Could you check a few things on this drawing? It's one solid part, dimensions in mm from its lowest x, y, z. A direction names the side the tool comes from. Round coordinates to 2 decimals unless told otherwise and drop trailing zeros. Loops run counter-clockwise (first coordinate to the right, second up) from the corner with the lowest first, then second, coordinate; pieces in that order, holes last. Notation, with made-up numbers: (53.25, 86.5) -> (83.25, 86.5) arc R36 cw to (83.25, 121.5) -> close; hole circle Ø11 at (25.5, 81.25). An arc over 180 degrees is marked (long way). Use one line per item in the form item = value. Start each with the question number.
Item 1: For the marked faces 1 and 2, which set-ups out of +Z, -Z, +X, -X, +Y, -Y let a thin tool reach every point of the face, with its end or its side?
Item 2: If I drill on L1, parallel to Z at x = 550, y = 694.5; L2, parallel to Z at x = 361, y = 277 (1 decimal); L3, parallel to Y at x = 428, z = 458 (1 decimal), over which ranges is the centre line in solid material (lowest first)? Write a range as [from, to].
Item 3: If we section it at B-B (z = 282.5): Write out the boundary of the cut face in (x, y) (1 decimal).
Item 4: I'm going to push flat-ended pins straight in: pin 1 Ø3 at (x, z) = (148, 293.5) entering from -Y (1 decimal); pin 2 Ø6 at (x, z) = (396, 549) entering from +Y; pin 3 Ø10 at (y, z) = (592, 236) entering from -X. Where does each tip first touch, or does it pass through?
Item 5: If we section it at A-A (z = 608): Write out the boundary of the cut face in (x, y) (1 decimal).
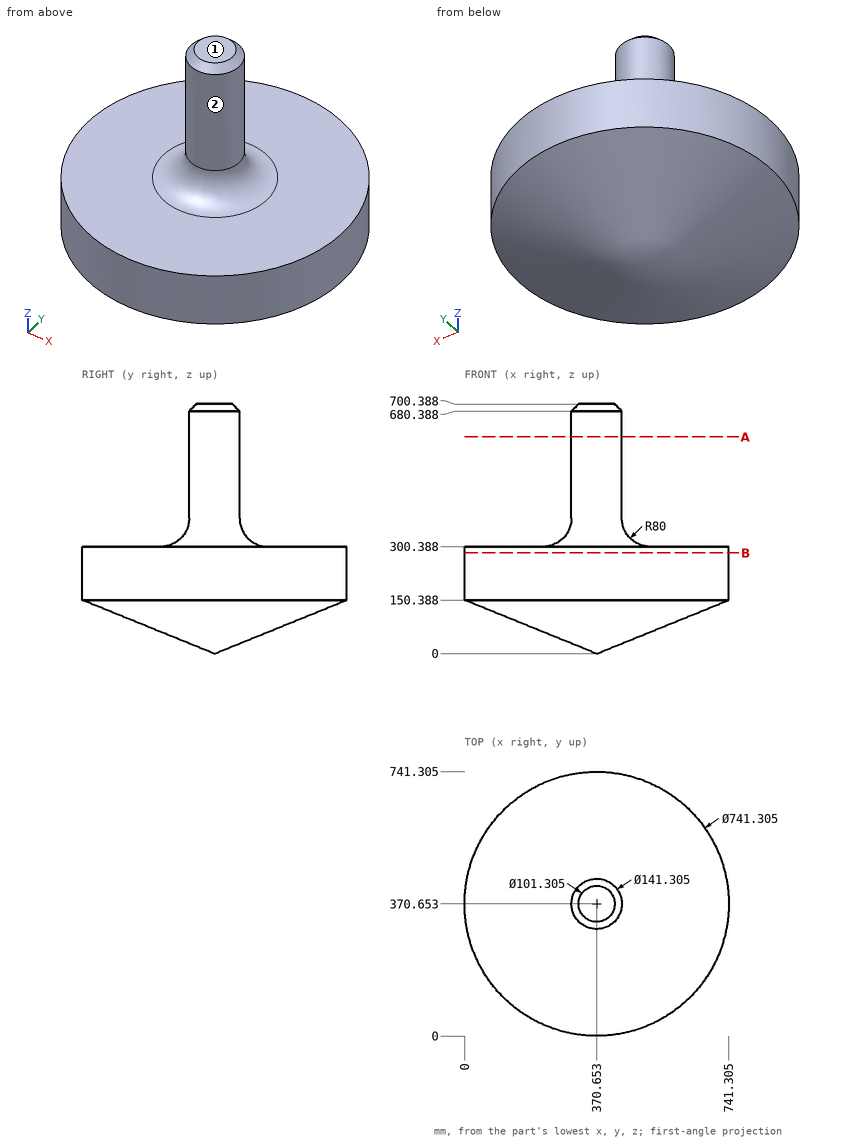
Values found:
q1.face_1 = +Z, +X, -X, +Y, -Y
q1.face_2 = +Z
q2.L1 = [150.2, 300.39]
q2.L2 = [38.2, 323.8]
q2.L3 = [329.4, 411.9]
q3.outline = circle Ø741.3 at (370.7, 370.7)
q4.pin_1 = 73.2
q4.pin_2 = 437.68
q4.pin_3 = 69.69
q5.outline = circle Ø141.3 at (370.7, 370.7)
